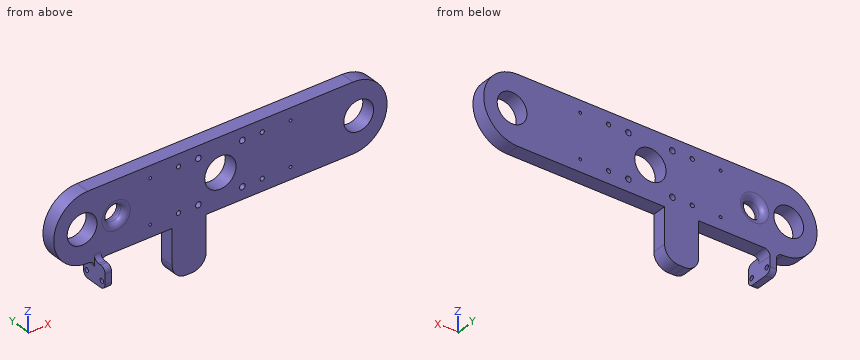
```python
from build123d import *

# Parameters (mm, degrees)
BOSS_EXTRUDE1_DEPTH = 10
SKETCH2_R           = 10.5
SKETCH2_R_2         = 6
SKETCH2_R_3         = 11.05
SKETCH2_R_4         = 2
SKETCH2_R_5         = 1.5
SKETCH2_R_6         = 1
CUT_EXTRUDE1_DEPTH  = 10
FILLET1_R           = 4
FILLET2_R           = 4
SKETCH3_W           = 4.58
SKETCH3_H           = 20
BOSS_EXTRUDE2_DEPTH = 15
FILLET3_R           = 4
FILLET4_R           = 4
FILLET5_R           = 4
SKETCH4_R           = 1.6
CUT_EXTRUDE2_DEPTH  = 15


with BuildPart() as part:
    # Sketch1 → Boss-Extrude1 (new body)
    with BuildSketch(Plane(origin=(0, 0, 0), x_dir=(1, 0, 0), z_dir=(0, 1, 0))):
        with BuildLine():
            Line((-34, 49), (-34, 24))
            Line((-34, 24), (-10, 24))
            Line((-10, 24), (-10, 49))
            ThreePointArc((-10, 49), (-12.928932188, 56.071067812), (-20, 59))
            Line((-20, 59), (-24, 59))
            ThreePointArc((-24, 59), (-31.071067812, 56.071067812), (-34, 49))
        make_face()
        with BuildLine():
            Line((-93.5, -24), (93.5, -24))
            ThreePointArc((93.5, -24), (117.5, 0), (93.5, 24))
            Line((93.5, 24), (-93.5, 24))
            ThreePointArc((-93.5, 24), (-117.5, 0), (-93.5, -24))
        make_face()
    extrude(amount=BOSS_EXTRUDE1_DEPTH)

    # Sketch2 → Cut-Extrude1 (cut)
    with BuildSketch(Plane(origin=(0, 10, 0), x_dir=(1, 0, 0), z_dir=(0, 1, 0))):
        with Locations(Location((-97.5, 0, 0), (0, 0, 270))):
            Circle(SKETCH2_R)
        with Locations(Location((97.5, 0, 0), (0, 0, 270))):
            Circle(SKETCH2_R)
        with Locations(Location((-73.5, 0, 0), (0, 0, 270))):
            Circle(SKETCH2_R_2)
        with Locations(Location((0, 0, 0), (0, 0, 270))):
            Circle(SKETCH2_R_3)
        with Locations(Location((-15.5, 15.5, 0), (0, 0, 270))):
            Circle(SKETCH2_R_4)
        with Locations(Location((15.5, 15.5, 0), (0, 0, 270))):
            Circle(SKETCH2_R_4)
        with Locations(Location((-15.5, -15.5, 0), (0, 0, 270))):
            Circle(SKETCH2_R_4)
        with Locations(Location((15.5, -15.5, 0), (0, 0, 270))):
            Circle(SKETCH2_R_4)
        with Locations(Location((29.5, 15.5, 0), (0, 0, 270))):
            Circle(SKETCH2_R_5)
        with Locations(Location((29.5, -15.5, 0), (0, 0, 270))):
            Circle(SKETCH2_R_5)
        with Locations(Location((-29.5, 15.5, 0), (0, 0, 270))):
            Circle(SKETCH2_R_5)
        with Locations(Location((-29.5, -15.5, 0), (0, 0, 270))):
            Circle(SKETCH2_R_5)
        with Locations(Location((-49.5, 15.5, 0), (0, 0, 270))):
            Circle(SKETCH2_R_6)
        with Locations(Location((-49.5, -15.5, 0), (0, 0, 270))):
            Circle(SKETCH2_R_6)
        with Locations(Location((49.5, 15.5, 0), (0, 0, 270))):
            Circle(SKETCH2_R_6)
        with Locations(Location((49.5, -15.5, 0), (0, 0, 270))):
            Circle(SKETCH2_R_6)
    extrude(amount=-CUT_EXTRUDE1_DEPTH, mode=Mode.SUBTRACT)

    # Fillet1
    fillet1_edges = [part.edges().sort_by_distance(p)[0] for p in [
        (-73.5, 10, -6),
    ]]
    fillet(fillet1_edges, radius=FILLET1_R)

    # Fillet2
    fillet2_edges = [part.edges().sort_by_distance(p)[0] for p in [
        (-73.5, 0, -6),
    ]]
    fillet(fillet2_edges, radius=FILLET2_R)

    # Sketch3 → Boss-Extrude2 (add)
    with BuildSketch(Plane(origin=(0, 0, -24), x_dir=(-1, 0, 0), z_dir=(0, 0, -1))):
        with Locations((86.62, 0)):
            Rectangle(SKETCH3_W, SKETCH3_H)
    extrude(amount=BOSS_EXTRUDE2_DEPTH)

    # Fillet3
    fillet3_edges = [part.edges().sort_by_distance(p)[0] for p in [
        (-86.62, 0, -24),
    ]]
    fillet(fillet3_edges, radius=FILLET3_R)

    # Fillet4
    fillet4_edges = [part.edges().sort_by_distance(p)[0] for p in [
        (-84.33, 5, -24),
        (-88.91, 5, -24),
    ]]
    fillet(fillet4_edges, radius=FILLET4_R)

    # Fillet5
    fillet5_edges = [part.edges().sort_by_distance(p)[0] for p in [
        (-86.62, -10, -24),
        (-86.62, -10, -39),
        (-86.62, 10, -39),
    ]]
    fillet(fillet5_edges, radius=FILLET5_R)

    # Sketch4 → Cut-Extrude2 (cut)
    with BuildSketch(Plane.ZY.offset(88.91)):
        with Locations((-34, 7)):
            Circle(SKETCH4_R)
        with Locations((-34, -7)):
            Circle(SKETCH4_R)
    extrude(amount=-CUT_EXTRUDE2_DEPTH, mode=Mode.SUBTRACT)


solid = part.part
```
Design review of the part built by this model. Coordinates are the model's own, in mm. Give positions to 0.01 mm unless a question says otherwise; leave off trailing zeros. Write each loop counter-clockwise with the first axis right and the second up, starting at its lowest first coordinate (ties: lowest second). Pieces come first, ordered by that corner, then holes. Notation, with made-up numbers: (-7, -21.75) - (22, -21.75) arc R11 ccw to (22, -5.75) - close; hole circle Ø11 at (37.25, -36.75). An arc over 180 degrees is marked (long way). Return JSON: item names as keys, results as strings. Group by question number.
(1) Insertion check: pin 1 (0.5 mm diameter, centred on x = -93, y = 7, fed in from -Z); pin 2 (8 mm diameter, centred on y = 3, z = -38, fed in from +X); pin 3 (1.6 mm diameter, centred on x = -86.5, y = -5.5, fed in from +Z); pin 4 (8 mm diameter, centred on x = -5, z = -25.5, fed in from +Y). Each pin has a flat end and moves straight along its axis. Give the tip position at first contact, or say it passes through.
(2) We need section B-B, the plane x = -73.5. Give the boundary of the cut face in (y, z), then the cut area to 3 significant figures.
(3) To check wall thickness, follow probe 1 along Y at (x, z) = (-86.15, -34); probe 2 along X at (y, z) = (1.5, -8); probe 3 along Y at (x, z) = (99, -20.5). State the ranges of each line that lie inside material, in increasing order.
(4) We need section C-C, the plane x = -97.5. Give the boundary of the cut face in (y, z).
(5) We need section A-A, the plane z = 0. Give the boundary of the cut face in (x, y), then the cut area to 3 significant figures.
(6) We need section D-D, the plane z = -53. Give the boundary of the cut face in (x, y).
Reported:
{
 "1": {"pin 1": "stops at z = -24", "pin 2": "stops at x = -10", "pin 3": "stops at z = -24", "pin 4": "stops at y = 10"},
 "2": {"outline": "(0, -24) - (10, -24) - (10, -10) arc R4 ccw to (6, -6) - (4, -6) arc R4 ccw to (0, -10) - close; (0, 10) arc R4 ccw to (4, 6) - (6, 6) arc R4 ccw to (10, 10) - (10, 24) - (0, 24) - close", "area": "346 mm2"},
 "3": {"probe 1": "y = -10 to -8.6, -5.4 to 5.4, 8.6 to 10", "probe 2": "x = -116.13 to -104.3, -90.7 to -7.62, 7.62 to 90.7, 104.3 to 116.13", "probe 3": "y = 0 to 10"},
 "4": {"outline": "(0, -23.66) - (10, -23.66) - (10, -10.5) - (0, -10.5) - close; (0, 10.5) - (10, 10.5) - (10, 23.66) - (0, 23.66) - close"},
 "5": {"outline": "(-117.5, 0) - (-108, 0) - (-108, 10) - (-117.5, 10) - close; (-87, 0) - (-83.5, 0) arc R4 ccw to (-79.5, 4) - (-79.5, 6) arc R4 ccw to (-83.5, 10) - (-87, 10) - close; (-67.5, 4) arc R4 ccw to (-63.5, 0) - (-11.05, 0) - (-11.05, 10) - (-63.5, 10) arc R4 ccw to (-67.5, 6) - close; (11.05, 0) - (87, 0) - (87, 10) - (11.05, 10) - close; (108, 0) - (117.5, 0) - (117.5, 10) - (108, 10) - close", "area": "1,580 mm2"},
 "6": {"outline": "(-33.17, 0) - (-10.83, 0) - (-10.83, 10) - (-33.17, 10) - close"}
}
